Geometry check sheet. Reference: drawing and pictorial views, mm from the part's lowest x, y, z. A direction names the side the tool comes from. Give positions to 0.01 mm unless a question says otherwise; leave off trailing zeros. Write each loop counter-clockwise with the first axis right and the second up, starting at its lowest first coordinate (ties: lowest second). Pieces come first, ordered by that corner, then holes. Notation, with made-up numbers: (24, 64) -> (38, 64) arc R15 cw to (38, 88) -> close; hole circle Ø11 at (-2, -31). An arc over 180 degrees is marked (long way). Answer as CSV lines item,"result".
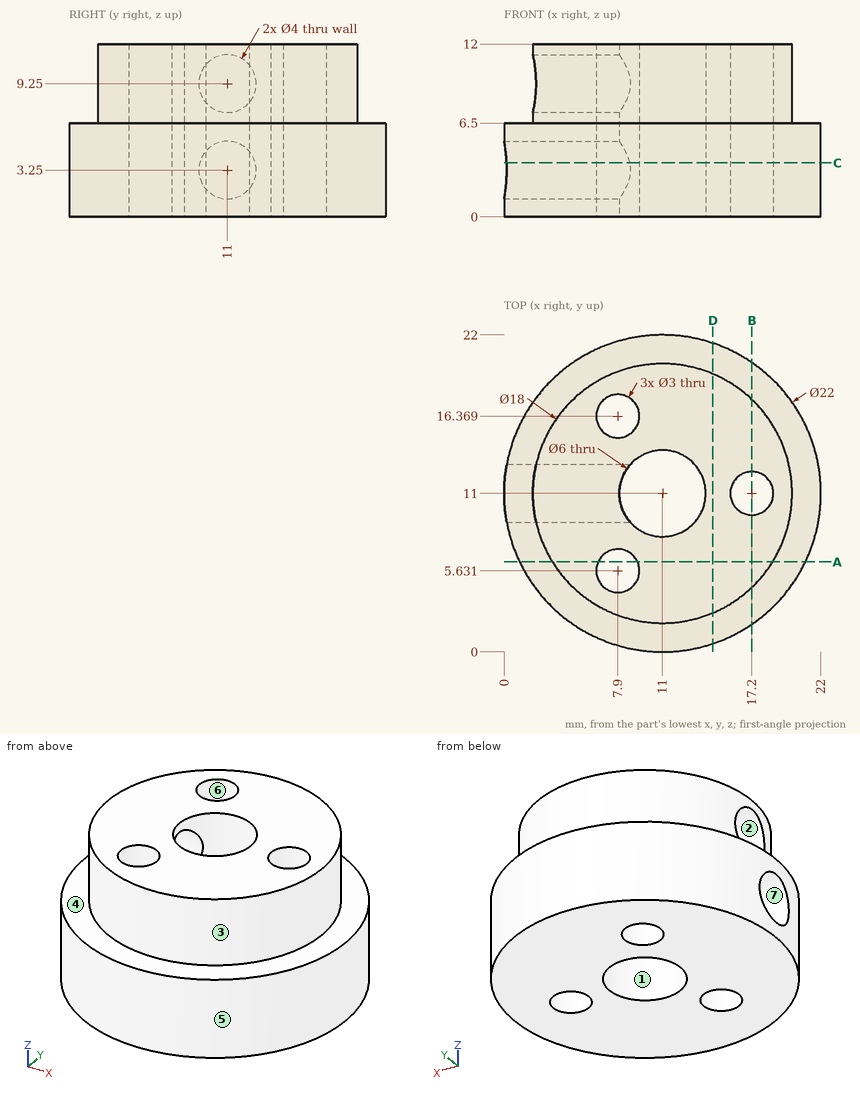
1) Section check D-D (x = 14.5). Record the boundary of the cut face in (y, z).
Reported:
outline,"(0.57, 0) -> (21.43, 0) -> (21.43, 6.5) -> (19.29, 6.5) -> (19.29, 12) -> (2.71, 12) -> (2.71, 6.5) -> (0.57, 6.5) -> close"
2) Draft check along Y on the marked faces 4, 5, 6 and 7. Enter one of: +Y half, -Y half, draft (parallel to the pull), parting line (faces both ways), or undercut.
Reported:
face 4,"draft"
face 5,"parting line"
face 6,"undercut"
face 7,"undercut"
3) Depth check by flat-ended pin: pin 1 (5 mm diameter, centred on y = 11, z = 9.25, fed in from -X); pin 2 (3.5 mm diameter, centred on x = 7.9, y = 16.37, fed in from -Z); pin 3 (3 mm diameter, centred on x = 18.5, z = 10, fed in from -Y); pin 4 (3 mm diameter, centred on y = 11, z = 3.25, fed in from -X). Enter the tip coordinate at first touch or a pass-through.
Reported:
pin 1,"x = 2"
pin 2,"z = 0"
pin 3,"y = 4.29"
pin 4,"x = 13.6"
4) Section check C-C (z = 3.75). Record the boundary of the cut face in (x, y), and give its area (3 significant figures).
Reported:
outline,"(0.17, 9.06) arc R11 ccw (long way) to (0.17, 12.94) -> (8.71, 12.94) arc R3 cw (long way) to (8.71, 9.06) -> close; hole circle Ø3 at (7.9, 5.63); hole circle Ø3 at (7.9, 16.37); hole circle Ø3 at (17.2, 11)"
area,"299 mm²"
5) Tool access check on the marked faces 1, 2 and 3. Record the directions out of +Z, -Z, +X, -X, +Y, -Y that give a thin tool (end or side, any length) a straight path to the whole face; none if there is none.
Reported:
face 1,"+Z, -Z"
face 2,"-X"
face 3,"+Z"
6) Section check A-A (y = 6.25). Record the boundary of the cut face in (x, z) (1 decimal).
Reported:
outline,"(1.1, 0) -> (6.5, 0) -> (6.5, 12) -> (3.4, 12) -> (3.4, 6.5) -> (1.1, 6.5) -> close; (9.3, 0) -> (20.9, 0) -> (20.9, 6.5) -> (18.6, 6.5) -> (18.6, 12) -> (9.3, 12) -> close"
7) Scan lines: line 1 along Z through (x, y) = (3, 10); line 2 along Z through (x, y) = (14.5, 20); line 3 along X through (y, z) = (12.75, 0.5) (1 decimal). Record each from-to range of solid material in increasing order.
Reported:
line 1,"0 to 1.52, 4.98 to 7.52, 10.98 to 12"
line 2,"0 to 6.5"
line 3,"0.1 to 8.6, 13.4 to 21.9"
8) Section check B-B (x = 17.2). Record the boundary of the cut face in (y, z), and give its area (3 significant figures).
Reported:
outline,"(1.91, 0) -> (9.5, 0) -> (9.5, 12) -> (4.48, 12) -> (4.48, 6.5) -> (1.91, 6.5) -> close; (12.5, 0) -> (20.09, 0) -> (20.09, 6.5) -> (17.52, 6.5) -> (17.52, 12) -> (12.5, 12) -> close"
area,"154 mm²"
